Can you work these out from the model? Positions are in its coordinate system, mm. Coordinates: 2 decimals unless noted, no trailing zeros. Write each loop counter-clockwise with the first axis right and the second up, starting at its lowest first coordinate (ties: lowest second). Pieces come first, ordered by that corner, then holes. Notation, with made-up numbers: (-1.5, -23) -> (28.5, -23) arc R11 cw to (28.5, -16) -> close; hole circle Ø10 at (79.5, 83.5). An arc over 180 degrees is marked (long way). Answer as CSV lines item,"result". Start each with the question number.
```python
from build123d import *

# Parameters (mm, degrees)
BOSS_EXTRUDE1_DEPTH = 1.25
SKETCH2_R           = 1.5
CUT_EXTRUDE1_DEPTH  = 10
SKETCH3_R           = 1
CUT_EXTRUDE2_DEPTH  = 10


with BuildPart() as part:
    # Sketch1 → Boss-Extrude1 (new, symmetric)
    with BuildSketch(Plane.XY):
        with BuildLine():
            Line((100, 6.15063129), (98.039215686, 22.030030676))
            ThreePointArc((98.039215686, 22.030030676), (14.786349801, 16.13665926), (-68.62745098, 18.949014823))
            Line((-68.62745098, 18.949014823), (-70, 3.007995119))
            ThreePointArc((-70, 3.007995119), (15.082076797, 0.139392445), (100, 6.15063129))
        make_face()
    extrude(amount=BOSS_EXTRUDE1_DEPTH, both=True)

    # Sketch2 → Cut-Extrude1 (cut, symmetric)
    with BuildSketch(Plane.XY):
        with Locations((0, 8)):
            Circle(SKETCH2_R)
    extrude(amount=CUT_EXTRUDE1_DEPTH, both=True, mode=Mode.SUBTRACT)

    # Sketch3 → Cut-Extrude2 (cut, symmetric)
    with BuildSketch(Plane.XY):
        with Locations((94, 13.486995845)):
            Circle(SKETCH3_R)
    extrude(amount=CUT_EXTRUDE2_DEPTH, both=True, mode=Mode.SUBTRACT)


solid = part.part
```
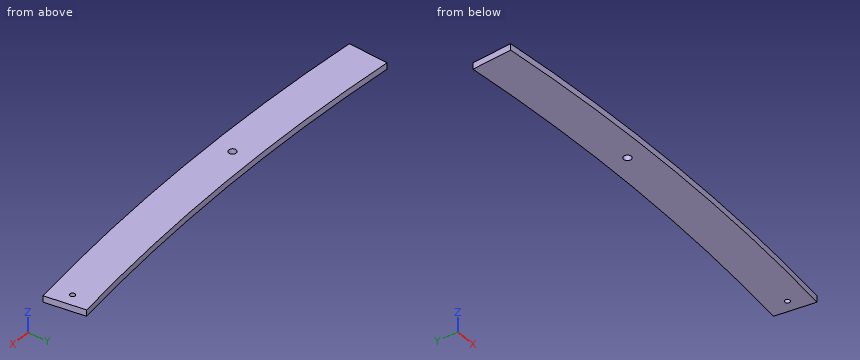
Q1. I need wall thicknesses on L1, parallel to Y at x = 94, z = 0.35; L2, parallel to X at y = 7, z = -1; L3, parallel to Y at x = 80.5, z = -0.9. Which ranges of each line are inside material? Lowest first, please.
Q2. Imagine slicing it at A-A (x = 0). Write out the boundary of the cut face in (y, z).
Q3. For pin 1 (1 mm diameter, centred on x = 41, z = 0, fed in from -Y), with a flat end and sliding along its axis, tell me the tip position at first contact or that it passes through.
Q4. Imagine slicing it at D-D (x = 70.5). Write out the boundary of the cut face in (y, z).
Q5. Imagine slicing it at B-B (y = 8). Write out the boundary of the cut face in (x, z), then the cut area to 3 significant figures.
Q6. Imagine slicing it at C-C (z = -0.3). Write out the boundary of the cut face in (x, y).
Entries:
1,L1,"5.43 to 12.49, 14.49 to 21.54"
1,L2,"-69.66 to -1.12, 1.12 to 99.9"
1,L3,"3.98 to 20.06"
2,outline,"(0, -1.25) -> (6.5, -1.25) -> (6.5, 1.25) -> (0, 1.25) -> close; (9.5, -1.25) -> (16, -1.25) -> (16, 1.25) -> (9.5, 1.25) -> close"
3,pin 1,"y = 1.01"
4,outline,"(3.05, -1.25) -> (19.11, -1.25) -> (19.11, 1.25) -> (3.05, 1.25) -> close"
5,outline,"(-69.57, -1.25) -> (-1.5, -1.25) -> (-1.5, 1.25) -> (-69.57, 1.25) -> close; (1.5, -1.25) -> (99.77, -1.25) -> (99.77, 1.25) -> (1.5, 1.25) -> close"
5,area,"416 mm2"
6,outline,"(-70, 3.01) arc R816 ccw to (100, 6.15) -> (98.04, 22.03) arc R800 cw to (-68.63, 18.95) -> close; hole circle Ø3 at (0, 8); hole circle Ø2 at (94, 13.49)"
